Part model, mm, in its own coordinate system. Give positions to 0.01 mm unless a question says otherwise; leave off trailing zeros. Order: outer loops, then holes, each group sorted by start corner. A loop starts at its lowest first (then second) coordinate and runs counter-clockwise, first axis right, second up. Notation, with made-up numbers: (14, -5) -> (28, -5) arc R30 cw to (28, 26) -> close; hole circle Ø6 at (-30, 66). An arc over 180 degrees is marked (long way). Write item = value, one per line. Start each with the question number.
Item 1: Band-saw the part on D-D on y = 28. Write the cut outline in (x, z), plus the area to 3 significant figures.
Item 2: Drill centre lines: line 1 along Y through (x, z) = (-6.35, 1.7); line 2 along Y through (x, z) = (6.35, 4); line 3 along X through (y, z) = (0, 1.7). Where is each one in solid material? Low to high.
Item 3: Band-saw the part on A-A on x = 6.35. Write the cut outline in (y, z).
Item 4: Flat gauge pins, fed straight in: P1, Ø5.5, axis at x = -6.35, y = 38.1, coming from the +Z side; P2, Ø5, axis at y = -16, z = 8.5, coming from the -X side; P3, Ø5, axis at x = 57, z = 15, coming from the -Y side (3 decimals). Where does each tip first touch, or does it go through?
Item 5: Band-saw the part on C-C on x = 50. Write the cut outline in (y, z), plus the area to 3 significant figures.
Item 6: Band-saw the part on B-B on z = 15.5. Write the cut outline in (x, y) (3 decimals), plus the area to 3 significant figures.
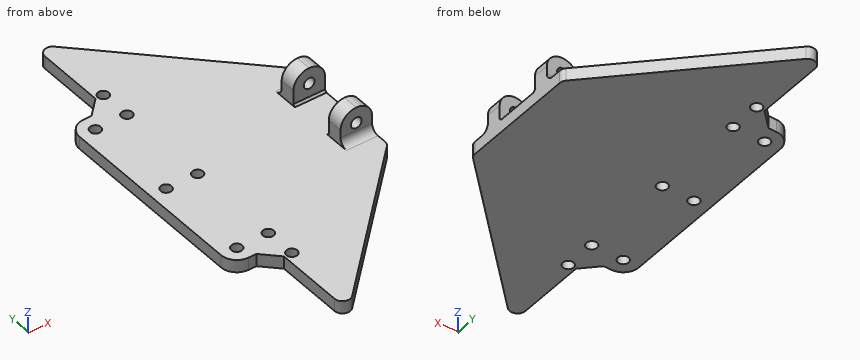
Autodesk Inventor part; units mm, degrees
ref_plane "YZ Plane" through (0, 0, 0) normal (1, 0, 0) x (0, 1, 0)
ref_plane "XZ Plane" through (0, 0, 0) normal (0, 1, 0) x (-1, 0, 0)
ref_plane "XY Plane" through (0, 0, 0) normal (0, 0, 1) x (1, 0, 0)
sketch "Sketch1" plane through (0, 0, 0) normal (0, 0, 1) x (1, 0, 0)
  line L0 (88.9, 0) -> (-12.7, 101.6)
  line L1 (-12.7, 101.6) -> (-12.7, -101.6)
  line L2 (-12.7, -101.6) -> (88.9, 0)
  line L3 (-12.7, 0) -> (88.9, 0)
  line L4 (64.73, 183.898) -> (-316.27, 183.898)
  line L5 (-316.27, 183.898) -> (-316.27, -183.898)
  line L6 (-316.27, -183.898) -> (64.73, -183.898)
  line L7 (64.73, -183.898) -> (64.73, 183.898)
  line L8 (64.73, 183.898) -> (-316.27, -183.898) construction
  line L9 (-316.27, 183.898) -> (64.73, -183.898) construction
  circle A0 centre (6.35, 38.1) radius 2.1844
  circle A1 centre (-6.35, 38.1) radius 2.1844
  circle A2 centre (-6.35, -38.1) radius 2.1844
  circle A3 centre (6.35, -38.1) radius 2.1844
  circle A4 centre (6.35, 0) radius 2.1844
  circle A5 centre (6.35, 88.9) radius 2.1844
  circle A6 centre (6.35, 50.8) radius 2.1844
  circle A7 centre (6.35, -50.8) radius 2.1844
  circle A8 centre (-6.35, 0) radius 2.1844
  circle A9 centre (-6.35, 38.1) radius 6.35
  circle A10 centre (-6.35, -38.1) radius 6.35
  line L10 (3.175, -85.725) -> (3.175, -44.45)
  line L11 (3.175, -44.45) -> (-11.204, -44.45)
  line L12 (-10.742, 44.45) -> (3.175, 44.45)
  line L13 (3.175, 44.45) -> (3.175, 85.725)
  point P0 (0, 0)
  point P1 (-125.77, 0)
  point P2 (64.73, 24.17)
  point P3 (-6.35, 44.45)
  point P4 (-12.7, 38.1)
  point P5 (-12.7, -38.1)
  point P6 (-6.35, -44.45)
  point P7 (64.73, -24.17)
  dimension "d0" = 101.6
  dimension "d2" = 381
  dimension "d4" = 12.7
  dimension "d5" = 12.7
  dimension "d6" = 3.175
  dimension "d7" = 3.175
extrude "Extrusion1" add sketch "Sketch1" along normal blind 5.08 contours L0 L7 L3 A4 A8 L1 A9 L12 L13 | A9 | L7 L2 L10 L11 A10 L1 L3 A8 A4 | A10
chamfer "Chamfer1" distance 6.35 angle 45 2 edges at (3.175, 44.45, 2.54) (3.175, -44.45, 2.54)
fillet "Fillet1" radius 3.175 4 edges at (3.175, 85.725, 2.54) (3.175, -85.725, 2.54) (64.73, 24.17, 2.54) (64.73, -24.17, 2.54)
sketch "Sketch2" plane through (0, 0, 5.08) normal (0, 0, 1) x (1, 0, 0)
  circle A0 centre (58.38, 0) radius 2.1844
  line L0 (58.38, 0) -> (0, 0) construction
  circle A1 centre (58.38, 12.7) radius 2.1844
  circle A2 centre (58.38, -12.7) radius 2.1844
  line L1 (58.38, 0) -> (58.38, -12.7) construction
  line L2 (64.73, -22.8548) -> (64.73, 22.8548) construction
  line L3 (52.03, -15.875) -> (64.73, -15.875)
  line L4 (64.73, -15.875) -> (64.73, -9.525)
  line L5 (64.73, -9.525) -> (52.03, -9.525)
  line L6 (52.03, -9.525) -> (52.03, -15.875)
  line L7 (52.03, -15.875) -> (64.73, -9.525) construction
  line L8 (64.73, -15.875) -> (52.03, -9.525) construction
  line L9 (52.03, 15.875) -> (64.73, 15.875)
  line L10 (64.73, 15.875) -> (64.73, 9.525)
  line L11 (64.73, 9.525) -> (52.03, 9.525)
  line L12 (52.03, 9.525) -> (52.03, 15.875)
  line L13 (52.03, 15.875) -> (64.73, 9.525) construction
  line L14 (64.73, 15.875) -> (52.03, 9.525) construction
  dimension "d14" = 4.3688
  dimension "d15" = 12.7
  dimension "d16" = 6.35
  dimension "d17" = 12.7
  dimension "d18" = 6.35
  dimension "d19" = 12.7
  dimension "d20" = 6.35
extrude "Extrusion2" add sketch "Sketch2" along normal blind 12.7 contours A1 | A2 | L6 L5 L4 L3 | L9 L10 L11 L12
fillet "Fillet2" radius 3.175 2 edges at (58.38, -15.875, 5.08) (58.38, 15.875, 5.08)
fillet "Fillet3" radius 6.35 4 edges at (64.73, -12.7, 17.78) (64.73, 12.7, 17.78) (52.03, 12.7, 17.78) (52.03, -12.7, 17.78)
sketch "Sketch3" plane through (52.03, -15.875, 8.255) normal (0, -1, 0) x (1, 0, 0)
  arc A0 (12.7, 3.175) -> (0, 3.175) centre (6.35, 3.175) ccw
  circle A1 centre (6.35, 3.175) radius 2.1844
  point P0 (-52.03, -8.255)
  dimension "d28" = 4.3688
extrude "Extrusion3" cut sketch "Sketch3" against normal through all
chamfer "Chamfer3" distance 0.7937 angle 45 2 edges at (58.38, -9.525, 5.08) (58.38, 9.525, 5.08)
properties part number "wedge"
Values found:
q1.outline = (-12.7, 0) -> (60.9, 0) -> (60.9, 5.08) -> (-12.7, 5.08) -> close
q1.area = 374 mm^2
q2.line_1 = -44.45 to -40.28, -35.92 to -2.18, 2.18 to 35.92, 40.28 to 44.45
q2.line_2 = -81.23 to -52.98, -48.62 to -40.28, -35.92 to -2.18, 2.18 to 35.92, 40.28 to 48.62, 52.98 to 81.23
q2.line_3 = -12.7 to -8.53, -4.17 to 4.17, 8.53 to 64.73
q3.outline = (-81.23, 0) -> (-52.98, 0) -> (-52.98, 5.08) -> (-81.23, 5.08) -> close; (-48.62, 0) -> (-40.28, 0) -> (-40.28, 5.08) -> (-48.62, 5.08) -> close; (-35.92, 0) -> (-2.18, 0) -> (-2.18, 5.08) -> (-35.92, 5.08) -> close; (2.18, 0) -> (35.92, 0) -> (35.92, 5.08) -> (2.18, 5.08) -> close; (40.28, 0) -> (48.62, 0) -> (48.62, 5.08) -> (40.28, 5.08) -> close; (52.98, 0) -> (81.23, 0) -> (81.23, 5.08) -> (52.98, 5.08) -> close
q4.P1 = 5.08
q4.P2 = 52.03
q4.P3 = -15.875
q5.outline = (-38.9, 0) -> (38.9, 0) -> (38.9, 5.08) -> (-38.9, 5.08) -> close
q5.area = 395 mm^2
q6.outline = (53.506, -15.875) -> (63.254, -15.875) -> (63.254, -9.525) -> (53.506, -9.525) -> close; (53.506, 9.525) -> (63.254, 9.525) -> (63.254, 15.875) -> (53.506, 15.875) -> close
q6.area = 124 mm^2
